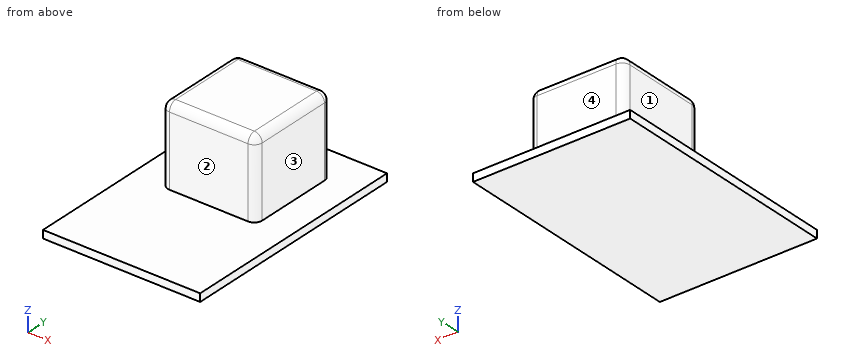
from build123d import *

# Parameters (mm, degrees)
SKETCH_1_W      = 200
SKETCH_1_H      = 300
EXTRUDE_1_DEPTH = 10
SKETCH_2_W      = 120
SKETCH_2_H      = 120
EXTRUDE_2_DEPTH = 100
FILLET_1_R      = 10


with BuildPart() as part:
    # 草图1 → 凸台-拉伸1 (new body)
    with BuildSketch(Plane.XY):
        Rectangle(SKETCH_1_W, SKETCH_1_H)
    extrude(amount=-EXTRUDE_1_DEPTH)

    # 草图2 → 凸台-拉伸2 (add)
    with BuildSketch(Plane.XY):
        with Locations((0, 50)):
            Rectangle(SKETCH_2_W, SKETCH_2_H)
    extrude(amount=EXTRUDE_2_DEPTH)

    # 圆角1
    fillet_1_edges = [part.edges().sort_by_distance(p)[0] for p in [
        (60, -10, 50),
        (60, 110, 50),
        (-60, 110, 50),
        (-60, -10, 50),
        (60, 50, 100),
        (0, 110, 100),
        (-60, 50, 100),
        (0, -10, 100),
    ]]
    fillet(fillet_1_edges, radius=FILLET_1_R)


solid = part.part
Here's how the part is built. I have some questions about the finished solid (model axes, mm). Face numbers are marked on the shaded views. A direction names the side the tool comes from. Round coordinates to 2 decimals unless told otherwise and drop trailing zeros. Write each loop counter-clockwise with the first axis right and the second up, starting at its lowest first coordinate (ties: lowest second). Pieces come first, ordered by that corner, then holes. Notation, with made-up numbers: (-17.5, 32) -> (-9.5, 32) arc R25 ccw to (-9.5, 68) -> close; hole circle Ø5 at (8.5, 79). An arc over 180 degrees is marked (long way). One line per item, written item: value.
1) For the marked faces 1, 2, 3 and 4, which set-ups out of +Z, -Z, +X, -X, +Y, -Y let a thin tool reach every point of the face, with its end or its side?
Filled sheet:
face 1: +Z, -X, +Y, -Y
face 2: +Z, +X, -X, -Y
face 3: +Z, +X, +Y, -Y
face 4: +Z, +X, -X, +Y
2) Suppose I cut it at B-B on z = 59. List the corners of the cut face in (x, y) for me.
Filled sheet:
outline: (-60, 0) arc R10 ccw to (-50, -10) -> (50, -10) arc R10 ccw to (60, 0) -> (60, 100) arc R10 ccw to (50, 110) -> (-50, 110) arc R10 ccw to (-60, 100) -> close
3) Suppose I cut it at D-D on x = -83. List the corners of the cut face in (y, z) for me.
Filled sheet:
outline: (-150, -10) -> (150, -10) -> (150, 0) -> (-150, 0) -> close
4) I'm going to push flat-ended pins straight in: pin 1 Ø2 at (x, y) = (-1.5, -28.5) entering from +Z; pin 2 Ø1 at (y, z) = (25, 47.5) entering from +X. Where does each tip first touch, or does it pass through?
Filled sheet:
pin 1: stops at z = 0
pin 2: stops at x = 60
5) Suppose I cut it at C-C on y = 44. List the corners of the cut face in (x, z) for me.
Filled sheet:
outline: (-100, -10) -> (100, -10) -> (100, 0) -> (60, 0) -> (60, 90) arc R10 ccw to (50, 100) -> (-50, 100) arc R10 ccw to (-60, 90) -> (-60, 0) -> (-100, 0) -> close
6) Suppose I cut it at A-A on x = -5. List the corners of the cut face in (y, z) for me, plus the area to 3 significant figures.
Filled sheet:
outline: (-150, -10) -> (150, -10) -> (150, 0) -> (110, 0) -> (110, 90) arc R10 ccw to (100, 100) -> (0, 100) arc R10 ccw to (-10, 90) -> (-10, 0) -> (-150, 0) -> close
area: 15,000 mm2
7) If I drill on line 1 (X direction, y = 41, z = 38); line 2 (Z direction, x = 13, y = -74); line 3 (Y direction, x = -49.5, z = 9.5), over which ranges is the centre line in solid material (lowest first)? Write a range as [from, to].
Filled sheet:
line 1: x = [-60, 60]
line 2: z = [-10, 0]
line 3: y = [-10, 110]
